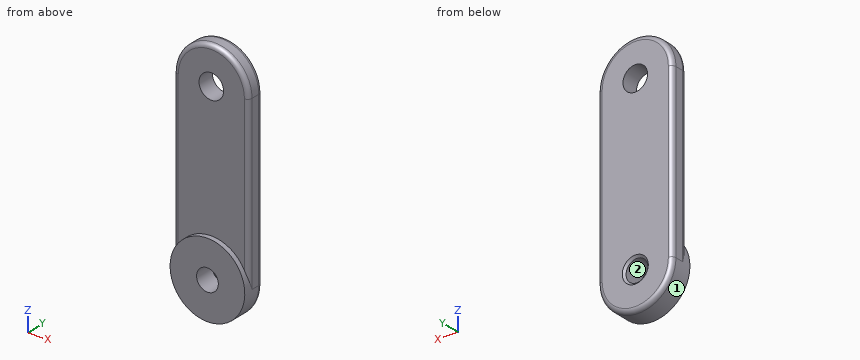
```python
from build123d import *
from build123d.topology import SkipClean

# Parameters (mm, degrees)
SKETCH1_R           = 2.55
SKETCH1_R_2         = 2.875
BOSS_EXTRUDE1_DEPTH = 4
BOSS_EXTRUDE2_START = 5
SKETCH3_R           = 8.75
SKETCH3_R_2         = 2.55
BOSS_EXTRUDE2_DEPTH = 5
FILLET2_R           = 1
SKETCH5_R           = 8.75
CUT_EXTRUDE2_DEPTH  = 3.84


with BuildPart() as part:
    # Sketch1 → Boss-Extrude1 (new body)
    with BuildSketch(Plane(origin=(0, 0, 0), x_dir=(1, 0, 0), z_dir=(0, 1, 0))):
        with BuildLine():
            Line((-8.75, 0), (-8.75, 40))
            ThreePointArc((-8.75, 40), (0, 48.75), (8.75, 40))
            Line((8.75, 40), (8.75, 0))
            ThreePointArc((8.75, 0), (0, -8.75), (-8.75, 0))
        make_face()
        with Locations(Location((0, 40, 0), (0, 0, 270))):
            Circle(SKETCH1_R, mode=Mode.SUBTRACT)
        with Locations(Location((0, 0, 0), (0, 0, 270))):
            Circle(SKETCH1_R_2, mode=Mode.SUBTRACT)
    extrude(amount=BOSS_EXTRUDE1_DEPTH)

    # Sketch3 → Boss-Extrude2 (add)
    with SkipClean():  # the faces are left unmerged after this step: merging them gives an invalid solid
        with BuildSketch(Plane.XZ.offset(BOSS_EXTRUDE2_START)):
            with Locations(Location((0, -40, 0), (0, 0, 270))):
                Circle(SKETCH3_R)
            with Locations(Location((0, -40, 0), (0, 0, 270))):
                Circle(SKETCH3_R_2, mode=Mode.SUBTRACT)
        extrude(amount=-BOSS_EXTRUDE2_DEPTH)

    # Fillet2
    # the kernel refuses this fillet: 1 mm, written as the material it takes off along each edge
    with BuildSketch(Plane(origin=(0, 4, -40), x_dir=(-1, 0, 0), z_dir=(0, 0, 1))) as fillet2_piece_1:
        with BuildLine():
            CenterArc((8.75 - FILLET2_R, FILLET2_R), FILLET2_R, 270, 90)
            Line((8.75 - FILLET2_R, 0), (8.75, 0))
            Line((8.75, 0), (8.75, FILLET2_R))
        make_face()
    revolve(axis=Axis((0, 4, -40), (0, -1, 0)), revolution_arc=180, mode=Mode.SUBTRACT)
    with BuildSketch(Plane(origin=(-8.75, 4, 0), x_dir=(1, 0, 0), z_dir=(0, 0, -1))) as fillet2_piece_2:
        with BuildLine():
            CenterArc((FILLET2_R, FILLET2_R), FILLET2_R, 180, 90)
            Line((0, FILLET2_R), (0, 0))
            Line((0, 0), (FILLET2_R, 0))
        make_face()
    extrude(amount=40, mode=Mode.SUBTRACT)
    with BuildSketch(Plane(origin=(0, -5, -40), x_dir=(0, 0, -1), z_dir=(-1, 0, 0))) as fillet2_piece_3:
        with BuildLine():
            CenterArc((8.75 - FILLET2_R, -FILLET2_R), FILLET2_R, 0, 90)
            Line((8.75 - FILLET2_R, 0), (8.75, 0))
            Line((8.75, 0), (8.75, -FILLET2_R))
        make_face()
    revolve(axis=Axis((0, -5, -40), (0, -1, 0)), mode=Mode.SUBTRACT)
    with BuildSketch(Plane(origin=(0, 4, 0), x_dir=(1, 0, 0), z_dir=(0, 0, -1))) as fillet2_piece_4:
        with BuildLine():
            CenterArc((8.75 - FILLET2_R, FILLET2_R), FILLET2_R, 270, 90)
            Line((8.75 - FILLET2_R, 0), (8.75, 0))
            Line((8.75, 0), (8.75, FILLET2_R))
        make_face()
    revolve(axis=Axis((0, 4, 0), (0, -1, 0)), revolution_arc=180, mode=Mode.SUBTRACT)
    with BuildSketch(Plane(origin=(-8.75, 0, 0), x_dir=(1, 0, 0), z_dir=(0, 0, -1))) as fillet2_piece_5_section:
        with BuildLine():
            CenterArc((FILLET2_R, -FILLET2_R), FILLET2_R, 90, 90)
            Line((0, -FILLET2_R), (0, 0))
            Line((0, 0), (FILLET2_R, 0))
        make_face()
    fillet2_piece_5 = extrude(amount=44.25, mode=Mode.PRIVATE)
    fillet2_piece_5 = fillet2_piece_5 - Plane(origin=(0, 0, -40), x_dir=(0, 0, -1), z_dir=(0, -1, 0)) * Cylinder(8.75, 93, mode=Mode.PRIVATE)
    add(fillet2_piece_5, mode=Mode.SUBTRACT)
    with BuildSketch(Plane(origin=(8.75, 0, -44.25), x_dir=(0, 1, 0), z_dir=(0, 0, 1))) as fillet2_piece_6_section:
        with BuildLine():
            CenterArc((FILLET2_R, FILLET2_R), FILLET2_R, 180, 90)
            Line((0, FILLET2_R), (0, 0))
            Line((0, 0), (FILLET2_R, 0))
        make_face()
    fillet2_piece_6 = extrude(amount=44.25, mode=Mode.PRIVATE)
    fillet2_piece_6 = fillet2_piece_6 - Plane(origin=(0, 0, -40), x_dir=(0, 0, -1), z_dir=(0, -1, 0)) * Cylinder(8.75, 93, mode=Mode.PRIVATE)
    add(fillet2_piece_6, mode=Mode.SUBTRACT)
    with BuildSketch(Plane(origin=(0, 0, 0), x_dir=(1, 0, 0), z_dir=(0, 0, -1))) as fillet2_piece_7:
        with BuildLine():
            CenterArc((8.75 - FILLET2_R, -FILLET2_R), FILLET2_R, 0, 90)
            Line((8.75 - FILLET2_R, 0), (8.75, 0))
            Line((8.75, 0), (8.75, -FILLET2_R))
        make_face()
    revolve(axis=Axis((0, 0, 0), (0, -1, 0)), revolution_arc=180, mode=Mode.SUBTRACT)
    with BuildSketch(Plane(origin=(8.75, 4, -40), x_dir=(0, -1, 0), z_dir=(0, 0, 1))) as fillet2_piece_8:
        with BuildLine():
            CenterArc((FILLET2_R, -FILLET2_R), FILLET2_R, 90, 90)
            Line((0, -FILLET2_R), (0, 0))
            Line((0, 0), (FILLET2_R, 0))
        make_face()
    extrude(amount=40, mode=Mode.SUBTRACT)

    # Chamfer1: read off the stored shape, not the designer's step
    # Chamfer1 outline → Chamfer1 (revolve, cut)
    with BuildSketch(Plane.XY.offset(-40)):
        Polygon((3.05, -5), (2.55, -4.5), (2.55, -5), align=None)
        Polygon((2.55, 4), (2.55, 3.5), (3.05, 4), align=None)
    revolve(axis=Axis((0, 0, -40), (0, 1, 0)), mode=Mode.SUBTRACT)

    # Sketch5 → Cut-Extrude2 (cut)
    with BuildSketch(Plane.XZ.offset(5)):
        with Locations(Location((0, -40, 0), (0, 0, 270))):
            Circle(SKETCH5_R)
    extrude(amount=-CUT_EXTRUDE2_DEPTH, mode=Mode.SUBTRACT)


solid = part.part
```
CAD build for the part. Positions are in the model's coordinates, mm. Face numbers are marked on the shaded views. A direction names the side the tool comes from. Coordinates: 2 decimals unless noted, no trailing zeros. Order: outer loops, then holes, each group sorted by start corner. A loop starts at its lowest first (then second) coordinate and runs counter-clockwise, first axis right, second up. Notation, with made-up numbers: (4.5, 86.25) - (62.5, 86.25) arc R23 ccw to (62.5, 107.25) - close; hole circle Ø2 at (-36, 54.5). An arc over 180 degrees is marked (long way). Answer in a Markdown table with one row per item.
1. Slice it at A-A, the plane z = -20. List the corners of the cut face in (x, y), then the cut area to 3 significant figures.
Answer:
| item | result |
|---|---|
| outline | (-8.75, 1) arc R1 ccw to (-7.75, 0) - (7.75, 0) arc R1 ccw to (8.75, 1) - (8.75, 3) arc R1 ccw to (7.75, 4) - (-7.75, 4) arc R1 ccw to (-8.75, 3) - close |
| area | 69.1 mm² |
2. Drill centre lines: L1, parallel to X at y = 0.5, z = -40; L2, parallel to Z at x = -1.25, y = 1.8; L3, parallel to Z at x = 0.75, y = 1.9. Where is each one in solid material? Low to high. Write a range as from..to.
Answer:
| item | result |
|---|---|
| L1 | -8.75..-2.55, 2.55..8.75 |
| L2 | -48.66..-42.22, -37.78..-2.59, 2.59..8.66 |
| L3 | -48.72..-42.44, -37.56..-2.78, 2.78..8.72 |
3. Flat gauge pin, fed straight in: P1, Ø9, axis at x = 0, z = 0, coming from the -Y side. Where does the tip first touch, or does it go through?
Answer:
| item | result |
|---|---|
| P1 | y = 0 |
4. 3-axis set-ups, long thin cutter, end or side, ignore diameter. For the marked faces 1 and 2: which of +Z, -Z, +X, -X, +Y, -Y reach the whole face in a straight line?
Answer:
| item | result |
|---|---|
| face 1 | -Y |
| face 2 | +Y, -Y |
